Read the model definition and answer for the solid it produces. Units are mm, in the model's axes. A direction names the side the tool comes from. Coordinates: 2 decimals unless noted, no trailing zeros. Loops run counter-clockwise (first coordinate to the right, second up) from the corner with the lowest first, then second, coordinate; pieces in that order, holes last. Notation, with made-up numbers: M 17,74 L 54,74 A26 cw 54,95 Z; hole C 46,-37 d3. An arc over 180 degrees is marked long. Use one line per item in the form item = value. Start each with the question number.
1. A tool of negligible diameter and unlimited length cuts with its end or side. For faces 4 (the flat face through (-20, 3, -1.57)), 5 (the flat face through (-20, 3, -6.37)), 6 (the flat face through (-38, 5, 24.94)), from which of +Z, -Z, +X, -X, +Y, -Y can it reach the whole face along a straight path? Write none if from no direction.
2. For a pull along Z with two mould halves and no side action, classify faces 1 (the flat face through (-31, 7.26, 7)), 2 (the cylindrical face through (-15.325, 3.232, -5.654)), 3 (the cylindrical face through (-39.137, 0.639, -13.077)) as released by +Z, released by -Z, zero draft, split by the parting line, or undercut.
3. Flat-ended cylindrical pins translate along their axes: pin 1 (2.5 mm diameter, centred on x = -18.5, z = -4, fed in from +Y); pin 2 (1.5 mm diameter, centred on x = -31.5, z = 9, fed in from +Y); pin 3 (1.5 mm diameter, centred on x = -30.5, y = 5.5, fed in from -Z). Find the tip coordinate at first contact, or state that the pin passes through.
4. Find the intervals of material crossed by probe 1 along X at (y, z) = (3.5, -0.5); probe 2 along X at (y, z) = (8, 1); probe 3 along Y at (x, z) = (5.5, 28), in increasing order. Write a range as [from, to].
5. The part is cut by section A-A (y = 3.75). Give the vertices of the cut face in (x, z).
6. The part is cut by section D-D (z = 28.5). Give the vertices of the cut face in (x, y).
7. The part is cut by section C-C (x = -19). Give the vertices of the cut face in (y, z), plus the area to 3 significant figures.
8. The part is cut by section B-B (z = 4). Give the vertices of the cut face in (x, y).
from build123d import *

# Parameters (mm, degrees)
SKETCH1_W           = 79
SKETCH1_H           = 49
BOSS_EXTRUDE1_DEPTH = 1.26
SKETCH2_R           = 1.65
CUT_EXTRUDE1_DEPTH  = 1.26
SKETCH3_W           = 5.27
SKETCH3_H           = 32.88
BOSS_EXTRUDE2_DEPTH = 8
SKETCH4_W           = 3
SKETCH4_H           = 20.4
BOSS_EXTRUDE3_DEPTH = 6
SKETCH5_W           = 11.5
SKETCH5_H           = 4.8
BOSS_EXTRUDE4_DEPTH = 4
FILLET1_R           = 2.5


with BuildPart() as part:
    # Sketch1 → Boss-Extrude1 (new body)
    with BuildSketch(Plane(origin=(0, 0, 0), x_dir=(1, 0, 0), z_dir=(0, 1, 0))):
        with Locations((-2.076516426, -7.930241605)):
            Rectangle(SKETCH1_W, SKETCH1_H)
    extrude(amount=BOSS_EXTRUDE1_DEPTH)

    # Sketch2 → Cut-Extrude1 (cut)
    with BuildSketch(Plane(origin=(0, 1.26, 0), x_dir=(1, 0, 0), z_dir=(0, 1, 0))):
        with Locations(Location((33.573483574, 12.719758395, 0), (0, 0, 270))):
            Circle(SKETCH2_R)
        with Locations(Location((33.573483574, -28.580241605, 0), (0, 0, 270))):
            Circle(SKETCH2_R)
        with Locations(Location((-37.526516426, -28.580241605, 0), (0, 0, 270))):
            Circle(SKETCH2_R)
        with Locations(Location((-37.526516426, 12.719758395, 0), (0, 0, 270))):
            Circle(SKETCH2_R)
    extrude(amount=-CUT_EXTRUDE1_DEPTH, mode=Mode.SUBTRACT)

    # Sketch3 → Boss-Extrude2 (add)
    with BuildSketch(Plane(origin=(0, 1.26, 0), x_dir=(1, 0, 0), z_dir=(0, 1, 0))):
        with Locations((-37.671516426, -8.500241605)):
            Rectangle(SKETCH3_W, SKETCH3_H)
    extrude(amount=BOSS_EXTRUDE2_DEPTH)

    # Sketch4 → Boss-Extrude3 (add)
    with BuildSketch(Plane(origin=(0, 1.26, 0), x_dir=(1, 0, 0), z_dir=(0, 1, 0))):
        with Locations((-31.076516426, -7.430241605)):
            Rectangle(SKETCH4_W, SKETCH4_H)
    extrude(amount=BOSS_EXTRUDE3_DEPTH)

    # Sketch5 → Boss-Extrude4 (add)
    with BuildSketch(Plane(origin=(0, 1.26, 0), x_dir=(1, 0, 0), z_dir=(0, 1, 0))):
        with Locations((-20.326516426, 3.969758395)):
            Rectangle(SKETCH5_W, SKETCH5_H)
    extrude(amount=BOSS_EXTRUDE4_DEPTH)

    # Fillet1
    # the kernel refuses this fillet: 2.5 mm, written as the material it takes off along each edge
    with BuildSketch(Plane(origin=(-26.076516426, 1.26, -6.369758395), x_dir=(0, 0, 1), z_dir=(0, 1, 0)), Plane(origin=(-26.076516426, 1.26, -1.569758395), x_dir=(1, 0, 0), z_dir=(0, 1, 0)), Plane(origin=(-14.576516426, 1.26, -1.569758395), x_dir=(0, 0, -1), z_dir=(0, 1, 0))) as fillet1_piece_1:
        with BuildLine():
            CenterArc((FILLET1_R, FILLET1_R), FILLET1_R, 180, 90)
            Line((0, FILLET1_R), (0, 0))
            Line((0, 0), (FILLET1_R, 0))
        make_face()
    extrude(amount=10.25, mode=Mode.SUBTRACT)
    with BuildSketch(Plane(origin=(-14.576516426, 1.26, -6.369758395), x_dir=(0, 0, 1), z_dir=(0, 1, 0))) as fillet1_piece_2:
        with BuildLine():
            CenterArc((FILLET1_R, -FILLET1_R), FILLET1_R, 90, 90)
            Line((0, -FILLET1_R), (0, 0))
            Line((0, 0), (FILLET1_R, 0))
        make_face()
    extrude(amount=10.25, mode=Mode.SUBTRACT)


solid = part.part
Computed values:
q1.face_4 = +Z, +X, +Y
q1.face_5 = -Z, +X, +Y
q1.face_6 = +Z, +X, -X, +Y
q2.face_1 = zero draft
q2.face_2 = released by -Z
q2.face_3 = undercut
q3.pin_1 = 5.26
q3.pin_2 = 7.26
q3.pin_3 = -2.77
q4.probe_1 = [-40.31, -35.04], [-32.58, -29.58]
q4.probe_2 = [-40.31, -35.04]
q4.probe_3 = [0, 1.26]
q5.outline = M -40.31,-7.94 L -35.04,-7.94 L -35.04,24.94 L -40.31,24.94 Z; M -32.58,-2.77 L -29.58,-2.77 L -29.58,17.63 L -32.58,17.63 Z; M -26.07,-3.97 A2.5 ccw -23.58,-6.37 L -17.08,-6.37 A2.5 ccw -14.58,-3.97 A2.5 ccw -17.08,-1.57 L -23.58,-1.57 A2.5 ccw Z
q6.outline = M -41.58,0 L -39.17,0 L -39.17,1.26 L -41.58,1.26 Z; M -35.88,0 L 31.93,0 L 31.93,1.26 L -35.88,1.26 Z; M 35.22,0 L 37.42,0 L 37.42,1.26 L 35.22,1.26 Z
q7.outline = M 0,-16.57 L 1.26,-16.57 L 1.26,-6.37 L 5.26,-6.37 L 5.26,-1.57 L 1.26,-1.57 L 1.26,32.43 L 0,32.43 Z
q7.area = 80.9 mm²
q8.outline = M -41.58,0 L 37.42,0 L 37.42,1.26 L -29.58,1.26 L -29.58,7.26 L -32.58,7.26 L -32.58,1.26 L -35.04,1.26 L -35.04,9.26 L -40.31,9.26 L -40.31,1.26 L -41.58,1.26 Z
